Here's the drawing with two shaded views (mm, measured from the low corner). I have some questions. A direction names the side the tool comes from. Coordinates: 2 decimals unless noted, no trailing zeros. Write each loop counter-clockwise with the first axis right and the second up, starting at its lowest first coordinate (ties: lowest second). Pieces come first, ordered by that corner, then holes. Notation, with made-up numbers: M 16,-26.5 L 54,-26.5 A22 cw 54,1.5 Z; hole C 28.25,-23.75 d1. An arc over 180 degrees is marked long. Use one line per item in the form item = value. Start each with the question number.
1. I want a section at D-D, the plane y = 60.5. List the corners of the cut face in (x, z) for me.
2. I want a section at A-A, the plane x = 21.5. List the corners of the cut face in (y, z) for me.
3. Thinking about a two-plate mould opening in X: for the marked faces 1, 2, 3 and 4, which applies, released by +X, released by -X, zero draft, split by the parting line, or undercut?
4. Please list where these lines run through material, in increasing order: line 1 along X through (y, z) = (111.5, 27.5); line 2 along Y through (x, z) = (15, 25); line 3 along Y through (x, z) = (21.5, 1.1). Write a range as [from, to].
5. On a 3-axis mill with a long thin cutter (end or side, diameter ignored), from which of +Z, -Z, +X, -X, +Y, -Y can I reach the whole of each face in a straight line? I mean the marked faces 5 and 6. Say none if no direction works.
6. I'm going to push flat-ended pins straight in: pin 1 Ø9.5 at (x, y) = (81.5, 76.5) entering from -Z; pin 2 Ø5 at (x, y) = (21.5, 76.5) entering from +Z. Where does each tip first touch, or does it pass through?
7. I want a section at B-B, the plane y = 76.5. List the corners of the cut face in (x, z) for me.
8. I want a section at C-C, the plane z = 27.5. List the corners of the cut face in (x, y) for me.
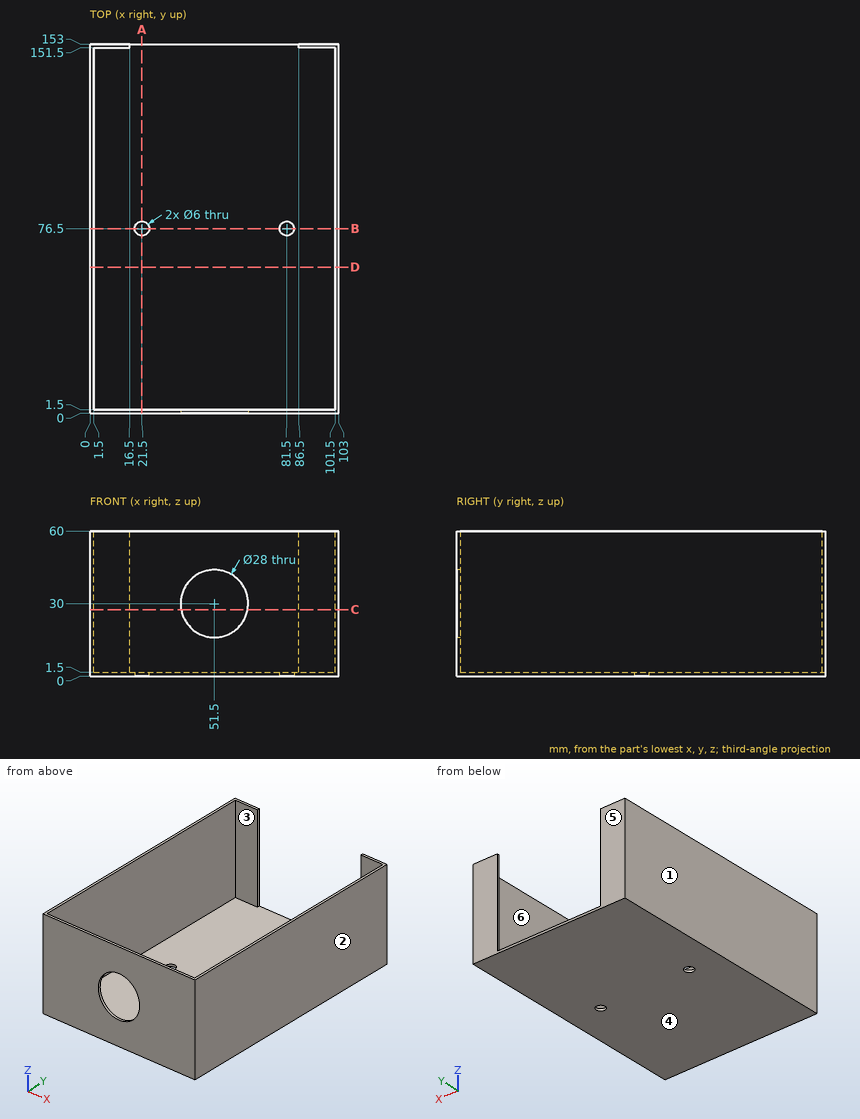
Answer list:
q1.outline = M 0,0 L 103,0 L 103,60 L 101.5,60 L 101.5,1.5 L 1.5,1.5 L 1.5,60 L 0,60 Z
q2.outline = M 0,0 L 73.5,0 L 73.5,1.5 L 1.5,1.5 L 1.5,60 L 0,60 Z; M 79.5,0 L 153,0 L 153,1.5 L 79.5,1.5 Z
q3.face_1 = released by -X
q3.face_2 = released by +X
q3.face_3 = undercut
q3.face_4 = zero draft
q4.line_1 = [0, 1.5], [101.5, 103]
q4.line_2 = [0, 1.5], [151.5, 153]
q4.line_3 = [0, 73.5], [79.5, 153]
q5.face_5 = +Z, -Z, +X, -X, +Y
q5.face_6 = +Z
q6.pin_1 = 0
q6.pin_2 = through
q7.outline = M 0,0 L 18.5,0 L 18.5,1.5 L 1.5,1.5 L 1.5,60 L 0,60 Z; M 24.5,0 L 78.5,0 L 78.5,1.5 L 24.5,1.5 Z; M 84.5,0 L 103,0 L 103,60 L 101.5,60 L 101.5,1.5 L 84.5,1.5 Z
q8.outline = M 0,0 L 37.73,0 L 37.73,1.5 L 1.5,1.5 L 1.5,151.5 L 16.5,151.5 L 16.5,153 L 0,153 Z; M 65.27,0 L 103,0 L 103,153 L 86.5,153 L 86.5,151.5 L 101.5,151.5 L 101.5,1.5 L 65.27,1.5 Z
